```python
from build123d import *

# Parameters (mm, degrees)
ESBO_O1_R                = 0.9
RESSALTO_EXTRUS_O1_DEPTH = 6


with BuildPart() as part:
    # Esbo_o1 → Ressalto-extrus_o1 (new body)
    with BuildSketch(Plane(origin=(0, 0, 0), x_dir=(1, 0, 0), z_dir=(0, 1, 0))):
        with BuildLine():
            Line((-0.036455066, 2.733587387), (0.036455066, 2.733587387))
            ThreePointArc((0.036455066, 2.733587387), (0.22673027, 2.657132964), (0.311206342, 2.470280816))
            Line((0.311206342, 2.470280816), (0.37, 1.088852607))
            ThreePointArc((0.37, 1.088852607), (0.393323165, 1.080646514), (0.416464521, 1.071940905))
            Line((0.416464521, 1.071940905), (1.349468012, 2.092384472))
            ThreePointArc((1.349468012, 2.092384472), (1.534286683, 2.181221351), (1.729189902, 2.117482292))
            Line((1.729189902, 2.117482292), (1.785042303, 2.070616563))
            ThreePointArc((1.785042303, 2.070616563), (1.88165761, 1.889742534), (1.826263789, 1.692305311))
            Line((1.826263789, 1.692305311), (0.983337409, 0.596278073))
            ThreePointArc((0.983337409, 0.596278073), (0.995929214, 0.575), (1.008060664, 0.55345614))
            Line((1.008060664, 0.55345614), (2.378711285, 0.73543818))
            ThreePointArc((2.378711285, 0.73543818), (2.577393846, 0.684692025), (2.685727696, 0.510583699))
            Line((2.685727696, 0.510583699), (2.698388408, 0.438781237))
            ThreePointArc((2.698388408, 0.438781237), (2.656136442, 0.238120569), (2.486792113, 0.122481344))
            Line((2.486792113, 0.122481344), (1.136560315, -0.175301598))
            ThreePointArc((1.136560315, -0.175301598), (1.132528916, -0.199695404), (1.127974019, -0.223996904))
            Line((1.127974019, -0.223996904), (2.294929112, -0.96562781))
            ThreePointArc((2.294929112, -0.96562781), (2.414509784, -1.132212308), (2.385583653, -1.33522268))
            Line((2.385583653, -1.33522268), (2.349128587, -1.398364706))
            ThreePointArc((2.349128587, -1.398364706), (2.187779513, -1.524920656), (1.98372277, -1.504653006))
            Line((1.98372277, -1.504653006), (0.757974019, -0.864855703))
            ThreePointArc((0.757974019, -0.864855703), (0.739205751, -0.88095111), (0.720095794, -0.896639307))
            Line((0.720095794, -0.896639307), (1.137324101, -2.214865816))
            ThreePointArc((1.137324101, -2.214865816), (1.121849759, -2.41934192), (0.969198506, -2.556263529))
            Line((0.969198506, -2.556263529), (0.900685394, -2.581200262))
            ThreePointArc((0.900685394, -2.581200262), (0.695736235, -2.574434559), (0.552447496, -2.427743491))
            Line((0.552447496, -2.427743491), (0.024723255, -1.149734213))
            ThreePointArc((0.024723255, -1.149734213), (0, -1.15), (-0.024723255, -1.149734213))
            Line((-0.024723255, -1.149734213), (-0.552447496, -2.427743491))
            ThreePointArc((-0.552447496, -2.427743491), (-0.695736235, -2.574434559), (-0.900685394, -2.581200262))
            Line((-0.900685394, -2.581200262), (-0.969198506, -2.556263529))
            ThreePointArc((-0.969198506, -2.556263529), (-1.121849759, -2.41934192), (-1.137324101, -2.214865816))
            Line((-1.137324101, -2.214865816), (-0.720095794, -0.896639307))
            ThreePointArc((-0.720095794, -0.896639307), (-0.739205751, -0.88095111), (-0.757974019, -0.864855703))
            Line((-0.757974019, -0.864855703), (-1.98372277, -1.504653006))
            ThreePointArc((-1.98372277, -1.504653006), (-2.187779513, -1.524920656), (-2.349128587, -1.398364706))
            Line((-2.349128587, -1.398364706), (-2.385583653, -1.33522268))
            ThreePointArc((-2.385583653, -1.33522268), (-2.414509784, -1.132212308), (-2.294929112, -0.96562781))
            Line((-2.294929112, -0.96562781), (-1.127974019, -0.223996904))
            ThreePointArc((-1.127974019, -0.223996904), (-1.132528916, -0.199695404), (-1.136560315, -0.175301598))
            Line((-1.136560315, -0.175301598), (-2.486792113, 0.122481344))
            ThreePointArc((-2.486792113, 0.122481344), (-2.656136442, 0.238120569), (-2.698388408, 0.438781237))
            Line((-2.698388408, 0.438781237), (-2.685727696, 0.510583699))
            ThreePointArc((-2.685727696, 0.510583699), (-2.577393846, 0.684692025), (-2.378711285, 0.73543818))
            Line((-2.378711285, 0.73543818), (-1.008060664, 0.55345614))
            ThreePointArc((-1.008060664, 0.55345614), (-0.995929214, 0.575), (-0.983337409, 0.596278073))
            Line((-0.983337409, 0.596278073), (-1.826263789, 1.692305311))
            ThreePointArc((-1.826263789, 1.692305311), (-1.88165761, 1.889742534), (-1.785042303, 2.070616563))
            Line((-1.785042303, 2.070616563), (-1.729189902, 2.117482292))
            ThreePointArc((-1.729189902, 2.117482292), (-1.534286683, 2.181221351), (-1.349468012, 2.092384472))
            Line((-1.349468012, 2.092384472), (-0.416464521, 1.071940905))
            ThreePointArc((-0.416464521, 1.071940905), (-0.393323165, 1.080646514), (-0.37, 1.088852607))
            Line((-0.37, 1.088852607), (-0.311206342, 2.470280816))
            ThreePointArc((-0.311206342, 2.470280816), (-0.22673027, 2.657132964), (-0.036455066, 2.733587387))
        make_face()
        with Locations(Location((0, 0, 0), (0, 0, 270))):
            Circle(ESBO_O1_R, mode=Mode.SUBTRACT)
    extrude(amount=RESSALTO_EXTRUS_O1_DEPTH)


solid = part.part
```
Geometry: final body of the model. Coordinates: model frame, mm. A direction names the side the tool comes from. Coordinates: 2 decimals unless noted, no trailing zeros. Order: outer loops, then holes, each group sorted by start corner. A loop starts at its lowest first (then second) coordinate and runs counter-clockwise, first axis right, second up. Notation, with made-up numbers: (27, 36.25) - (42, 36.25) arc R5 ccw to (42, 45.25) - close; hole circle Ø3 at (-27, 78). An arc over 180 degrees is marked (long way). Return JSON: item names as keys, results as strings. Group by question number.
1. Cut plane A-A (z = 0.45). Output: boundary loops of the cut face in (x, y), plus the area to 3 significant figures.
2. Pin query (flat end, axial travel): pin 1 (1.5 mm diameter, centred on x = -1.5, y = 1.5, fed in from -Z); pin 2 (1.5 mm diameter, centred on y = 5, z = 1, fed in from -X); pin 3 (1 mm diameter, centred on y = 3.5, z = -2, fed in from +X). Return the tip coordinate at first contact, or that it passes through.
3. Material intervals for line 1 along X through (y, z) = (0.5, -1.2); line 2 along X through (y, z) = (3.85, 1.1); line 3 along Z through (x, y) = (-1.75, 5.4), sorted ascending. Write a range as [from, to].
4. Cut plane B-B (x = -1.6). Output: boundary loops of the cut face in (y, z).
5. Cut plane C-C (x = 1.55). Output: boundary loops of the cut face in (y, z).
6. Set-up query: faces 5 (the face through (-0.93, 2.96, 1.56)), 6 (the face through (1, 6, -1)), 7 (the face through (-0.34, 2.96, -1.77)), 8 (the face through (-1.72, 2.96, 0.6)). Return all of +Z, -Z, +X, -X, +Y, -Y with unobstructed straight access to the full face (end or side cutting, diameter ignored); none if empty.
7. Pull-direction query (Z, two-part tool) for faces 1 (the face through (-1.4, 2.96, -1.14)), 2 (the face through (1.703, 2.958, 0.59)), 3 (the face through (-0.285, 2.958, 1.78)), 4 (the face through (1, 0, -1)); classes: pulls with the +Z half, pulls with the -Z half, needs draft (parallel to the pull), parting line crosses it, or undercut.
Resolved:
{
 "1": {"outline": "(-1.48, 0) - (-0.78, 0) - (-0.78, 6) - (-1.48, 6) - close; (0.78, 0) - (1.48, 0) - (1.48, 6) - (0.78, 6) - close", "area": "8.45 mm²"},
 "2": {"pin 1": "stops at z = -2.18", "pin 2": "stops at x = -2.42", "pin 3": "stops at x = 1.88"},
 "3": {"line 1": "x = [-1.45, -0.53], [-0.37, 0.37], [0.53, 1.45]", "line 2": "x = [-2.4, -1.21], [-0.78, 0.78], [1.21, 2.4]", "line 3": "z = [-2.1, -1.59], [-0.65, 0.04], [0.62, 1.38]"},
 "4": {"outline": "(0, -2.18) - (6, -2.18) - (6, -1.4) - (0, -1.4) - close; (0, -0.63) - (6, -0.63) - (6, 0.07) - (0, 0.07) - close; (0, 0.52) - (6, 0.52) - (6, 1.3) - (0, 1.3) - close"},
 "5": {"outline": "(0, -2.18) - (6, -2.18) - (6, -1.33) - (0, -1.33) - close; (0, -0.63) - (6, -0.63) - (6, 0.08) - (0, 0.08) - close; (0, 0.49) - (6, 0.49) - (6, 1.28) - (0, 1.28) - close"},
 "6": {"face 5": "+Y, -Y", "face 6": "+Z, -Z, +X, -X, +Y", "face 7": "-Z, +Y, -Y", "face 8": "-X, +Y, -Y"},
 "7": {"face 1": "undercut", "face 2": "undercut", "face 3": "pulls with the +Z half", "face 4": "needs draft"}
}
